Design review of the part built by this model. Coordinates are the model's own, in mm. Face numbers are marked on the shaded views. A direction names the side the tool comes from. Give positions to 0.01 mm unless a question says otherwise; leave off trailing zeros. Order: outer loops, then holes, each group sorted by start corner. A loop starts at its lowest first (then second) coordinate and runs counter-clockwise, first axis right, second up. Notation, with made-up numbers: M 66,15 L 89,15 A13 ccw 89,21 Z; hole C 49,85.5 d5. An arc over 180 degrees is marked long. Answer as a JSON object with one key per item and string values.
from build123d import *

# Parameters (mm, degrees)
BOSS_EXTRUDE1_DEPTH = 12.7
SKETCH2_R           = 7.100000009
SKETCH2_R_2         = 4.100000009
BOSS_EXTRUDE2_DEPTH = 3.499999906
SKETCH4_W           = 6.35
SKETCH4_H           = 6.35
BOSS_EXTRUDE4_DEPTH = 25.4
CIRPATTERN1_COUNT   = 3
SKETCH6_R           = 4.100000009
CUT_EXTRUDE1_DEPTH  = 39.1
SKETCH7_R           = 2.3
CUT_EXTRUDE2_DEPTH  = 5.7
CUT_EXTRUDE4_DEPTH  = 39.1


with BuildPart() as part:
    # Sketch1 → Boss-Extrude1 (new body)
    with BuildSketch(Plane(origin=(0, 0, 0), x_dir=(1, 0, 0), z_dir=(0, 1, 0))):
        Polygon((11.43, -19.797340731), (22.86, 0), (11.43, 19.797340731), (-11.43, 19.797340731), (-22.86, 0), (-11.43, -19.797340731), align=None)
    extrude(amount=BOSS_EXTRUDE1_DEPTH)

    # Sketch2 → Boss-Extrude2 (add)
    with BuildSketch(Plane.XZ):
        Circle(SKETCH2_R)
        Circle(SKETCH2_R_2, mode=Mode.SUBTRACT)
    extrude(amount=BOSS_EXTRUDE2_DEPTH)

    # Sketch4 → Boss-Extrude4 (add)
    with BuildSketch(Plane.XZ):
        Polygon((12.802528987, -3.725369347), (7.303267673, -0.550369347), (4.128267673, -6.049630662), (9.627528987, -9.224630662), align=None)
        with Locations((0, 9.775000009)):
            Rectangle(SKETCH4_W, SKETCH4_H)
        Polygon((-9.627528987, -9.224630662), (-4.128267673, -6.049630662), (-7.303267673, -0.550369347), (-12.802528987, -3.725369347), align=None)
    extrude(amount=BOSS_EXTRUDE4_DEPTH)

    # Sketch5 → Cut-Revolve1 (revolve, cut)
    with BuildSketch(Plane(origin=(0, 12.7, 0), x_dir=(1, 0, 0), z_dir=(0, 1, 0))):
        Polygon((0, -19.797340731), (0, -4.672340739), (-5, -4.672340739), (-5, -10.797340731), (-11.300000152, -10.797340731), (-11.300000152, -17.797340731), (-6.5, -17.797340731), (-6.5, -19.797340731), align=None)
    cut_revolve1 = revolve(axis=Axis((0, 12.7, 19.797340731), (0, 0, -1)), mode=Mode.SUBTRACT)

    # CirPattern1: Cut-Revolve1 ×3 about axis
    cirpattern1_axis = Axis((0, 0, 0), (0, 1, 0))
    for i in range(1, CIRPATTERN1_COUNT):
        add(cut_revolve1.rotate(cirpattern1_axis, i * 360 / CIRPATTERN1_COUNT), mode=Mode.SUBTRACT)

    # Sketch6 → Cut-Extrude1 (cut, through all)
    with BuildSketch(Plane(origin=(0, 12.7, 0), x_dir=(1, 0, 0), z_dir=(0, 1, 0))):
        Circle(SKETCH6_R)
    extrude(amount=-CUT_EXTRUDE1_DEPTH, mode=Mode.SUBTRACT)

    # Sketch7 → Cut-Extrude2 (cut)
    with BuildSketch(Plane(origin=(0, 12.7, 0), x_dir=(1, 0, 0), z_dir=(0, 1, 0))):
        with Locations((0, 10.16)):
            Circle(SKETCH7_R)
        with Locations((8.798818102, -5.08)):
            Circle(SKETCH7_R)
        with Locations((-8.798818102, -5.08)):
            Circle(SKETCH7_R)
    extrude(amount=-CUT_EXTRUDE2_DEPTH, mode=Mode.SUBTRACT)

    # Sketch9 → Cut-Extrude4 (cut, through all)
    with BuildSketch(Plane(origin=(0, 12.7, 0), x_dir=(1, 0, 0), z_dir=(0, 1, 0))):
        Polygon((-6.577186816, 19.797340731), (0, 16.000000152), (6.577186816, 19.797340731), align=None)
        Polygon((20.433593408, -4.202659497), (13.856406592, -8.000000076), (13.856406592, -15.594681234), align=None)
        Polygon((-13.856406592, -15.594681234), (-13.856406592, -8.000000076), (-20.433593408, -4.202659497), align=None)
    extrude(amount=-CUT_EXTRUDE4_DEPTH, mode=Mode.SUBTRACT)


solid = part.part
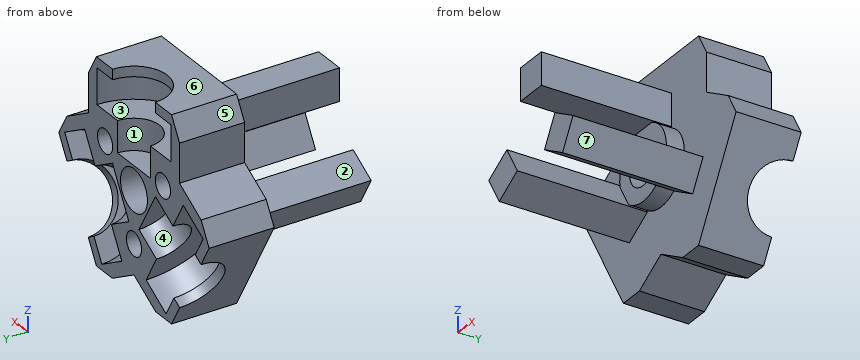
(1) To check wall thickness, follow L1, parallel to Z at x = 0, y = 10; L2, parallel to X at y = 4, z = 0; L3, parallel to X at y = 10.05, z = 5.08. State the ranges of each line that lie inside material, in increasing order. Write a range as from..to.
Checked values:
{"L1": "z = -16..-12.46, -7.86..-4.1, 4.1..4.67", "L2": "x = -22.86..-14.42, -12.47..-4.1, 4.1..12.47, 14.42..22.86", "L3": "x = -18.91..-11.1, -6.5..-4.24, 4.24..6.5, 11.1..18.91"}
(2) We need section A-A (y = -19.5). Write out the cut boundary in (x, z) (3 decimals).
Checked values:
{"outline": "M -12.803,-3.725 L -9.628,-9.225 L -4.128,-6.05 L -7.303,-0.55 Z; M -3.175,6.6 L 3.175,6.6 L 3.175,12.95 L -3.175,12.95 Z; M 4.128,-6.05 L 9.628,-9.225 L 12.803,-3.725 L 7.303,-0.55 Z"}
(3) We need section B-B (y = 2.5). Write out the cut boundary in (x, z), plus the area to 3 significant figures.
Checked values:
{"outline": "M -22.86,0 L -11.43,-19.8 L -6.58,-19.8 L 0,-16 L 6.58,-19.8 L 11.43,-19.8 L 22.86,0 L 20.43,4.2 L 13.86,8 L 13.86,15.59 L 11.43,19.8 L -11.43,19.8 L -13.86,15.59 L -13.86,8 L -20.43,4.2 Z; hole M -17.84,-4.69 L -12.98,-13.11 L -6.92,-9.61 L -11.78,-1.19 Z; hole M -4.86,10.8 L 4.86,10.8 L 4.86,17.8 L -4.86,17.8 Z; hole C 0,0 d8.2; hole M 6.92,-9.61 L 12.98,-13.11 L 17.84,-4.69 L 11.78,-1.19 Z", "area": "1,030 mm^2"}
(4) Tool access review of the marked faces 1, 2 and 3: name each direction out of +Z, -Z, +X, -X, +Y, -Y from which nothing blocks a thin tool from reaching the whole face with its end or side.
Checked values:
{"face 1": "+Z, +Y", "face 2": "+Z, -X, -Y", "face 3": "+Y"}
(5) Insertion check: pin 1 (3 mm diameter, centred on x = -9, z = 10.5, fed in from -Y); pin 2 (2.5 mm diameter, centred on x = -0.5, z = -10.5, fed in from +Y); pin 3 (8.5 mm diameter, centred on y = 7, z = 12.5, fed in from -X). Each pin has a flat end and moves straight along its axis. Give the tip position at first contact, or say it passes through.
Checked values:
{"pin 1": "stops at y = 0", "pin 2": "stops at y = 7", "pin 3": "stops at x = -13.86"}
(6) Draft analysis for pull direction X (two halves, no side actions). For the marked faces 4, 5, 6 and 7, state which applies: +X half, -X half, draft (parallel to the pull), parting line (faces both ways), or undercut.
Checked values:
{"face 4": "undercut", "face 5": "-X half", "face 6": "draft", "face 7": "+X half"}
